Check sheet for the modelled part. Datum: model origin and axes. Units: mm. A direction names the side the tool comes from. Round coordinates to 2 decimals unless told otherwise and drop trailing zeros. Loops run counter-clockwise (first coordinate to the right, second up) from the corner with the lowest first, then second, coordinate; pieces in that order, holes last. Notation, with made-up numbers: (48, -9.5) - (55, -9.5) arc R12 ccw to (55, 2.5) - close; hole circle Ø10 at (47.5, 35). An arc over 180 degrees is marked (long way). Answer in a Markdown table with one row per item. Add a question column.
(1) Cross-section at C-C on x = -12. Enter the section's corners in (y, z), then the cut area to 4 significant figures.
(2) Access from +Z, -Z, +X, -X, +Y, -Y to the whole of each face (thin tool, end or side, straight path). Record for faces 1 (the flat face through (-23, -13, 0)), 2 (the flat face through (10, -13, 50.8)).
(3) Cross-section at B-B on x = 16. Enter the section's corners in (y, z), then the cut area to 3 significant figures.
(4) Cross-section at A-A on y = -18.75. Enter the section's corners in (x, z) (1 decimal), then the cut area to 3 significant figures.
(5) Thickness scan on line 1 along X through (y, z) = (-4.25, 31); line 2 along X through (y, z) = (-18.25, 37); line 3 along X through (y, z) = (-13.75, -17.5). Record the ranges inside material, lowest first.
(6) Cross-section at D-D on z = -6. Enter the section's corners in (x, y), then the cut area to 3 significant figures.
(7) Gauge pin test, flat ends, axial feed: pin 1 (12 mm diameter, centred on y = -10.5, z = -12.5, fed in from -X); pin 2 (3 mm diameter, centred on x = -9, y = -3, fed in from -Z); pin 3 (3 mm diameter, centred on y = -5.5, z = -20.5, fed in from +X); pin 4 (2 mm diameter, centred on x = 5.5, z = 36.5, fed in from +Y). Record the tip position at first contact, or that the pin passes through.
from build123d import *

# Parameters (mm, degrees)
F0_W     = 40
F0_H     = 12.7
F0_W_2   = 14.2875
F0_H_2   = 28.575
F1_DEPTH = 25.4
F2_R     = 10
F3_R     = 5


with BuildPart() as f1:
    # F0 (on Front) → F1 (new body)
    with BuildSketch(Plane.XZ):
        with BuildLine():
            Line((14.2875, 29.925), (14.2875, 0))
            Line((14.2875, 0), (30.1625, 0))
            Line((30.1625, 0), (30.1625, 50.8))
            Line((30.1625, 50.8), (14.2875, 50.8))
            Line((14.2875, 50.8), (14.2875, 39.925))
            ThreePointArc((14.2875, 39.925), (17.823034, 38.460534), (19.2875, 34.925))
            ThreePointArc((19.2875, 34.925), (17.823034, 31.389466), (14.2875, 29.925))
        make_face()
        with BuildLine():
            Line((0, 12.7), (0, 0))
            Line((0, 0), (14.2875, 0))
            Line((14.2875, 0), (14.2875, 29.925))
            ThreePointArc((14.2875, 29.925), (9.2875, 34.925), (14.2875, 39.925))
            Line((14.2875, 39.925), (14.2875, 50.8))
            Line((14.2875, 50.8), (0, 50.8))
            Line((0, 50.8), (0, 12.7))
        make_face()
        Polygon((-40, 12.7), (0, 12.7), (0, 50.8), align=None)
        with Locations((-20, 6.35)):
            Rectangle(F0_W, F0_H)
        with Locations((7.14375, -14.2875)):
            Rectangle(F0_W_2, F0_H_2)
        Polygon((30.1625, 0), (14.2875, 0), (14.2875, -28.575), align=None)
    extrude(amount=F1_DEPTH)

    # F2
    f2_edges = [f1.edges().sort_by_distance(p)[0] for p in [
        (30.1625, -12.7, 50.8),
    ]]
    fillet(f2_edges, radius=F2_R)

    # F3
    f3_edges = [f1.edges().sort_by_distance(p)[0] for p in [
        (0, -12.7, 0),
    ]]
    fillet(f3_edges, radius=F3_R)


solid = f1.part
Answers:
| question | item | result |
|---|---|---|
| 1 | outline | (-25.4, 0) - (0, 0) - (0, 39.37) - (-25.4, 39.37) - close |
| 1 | area | 1,000 mm^2 |
| 2 | face 1 | -Z, -X, +Y, -Y |
| 2 | face 2 | +Z, +X, -X, +Y, -Y |
| 3 | outline | (-25.4, -25.49) - (0, -25.49) - (0, 30.23) - (-25.4, 30.23) - close; (-25.4, 39.62) - (0, 39.62) - (0, 50.8) - (-25.4, 50.8) - close |
| 3 | area | 1,700 mm^2 |
| 4 | outline | (-40, 0) - (-5, 0) arc R5 cw to (0, -5) - (0, -28.6) - (14.3, -28.6) - (30.2, 0) - (30.2, 40.8) arc R10 ccw to (20.2, 50.8) - (0, 50.8) - (-40, 12.7) - close; hole circle Ø10 at (14.3, 34.9) |
| 4 | area | 3,340 mm^2 |
| 5 | line 1 | x = -20.79 to 11.19, 17.38 to 30.16 |
| 5 | line 2 | x = -14.49 to 9.74, 18.84 to 30.16 |
| 5 | line 3 | x = 0 to 20.44 |
| 6 | outline | (0, -25.4) - (26.83, -25.4) - (26.83, 0) - (0, 0) - close |
| 6 | area | 681 mm^2 |
| 7 | pin 1 | stops at x = 0 |
| 7 | pin 2 | stops at z = 0 |
| 7 | pin 3 | stops at x = 19.61 |
| 7 | pin 4 | stops at y = 0 |
